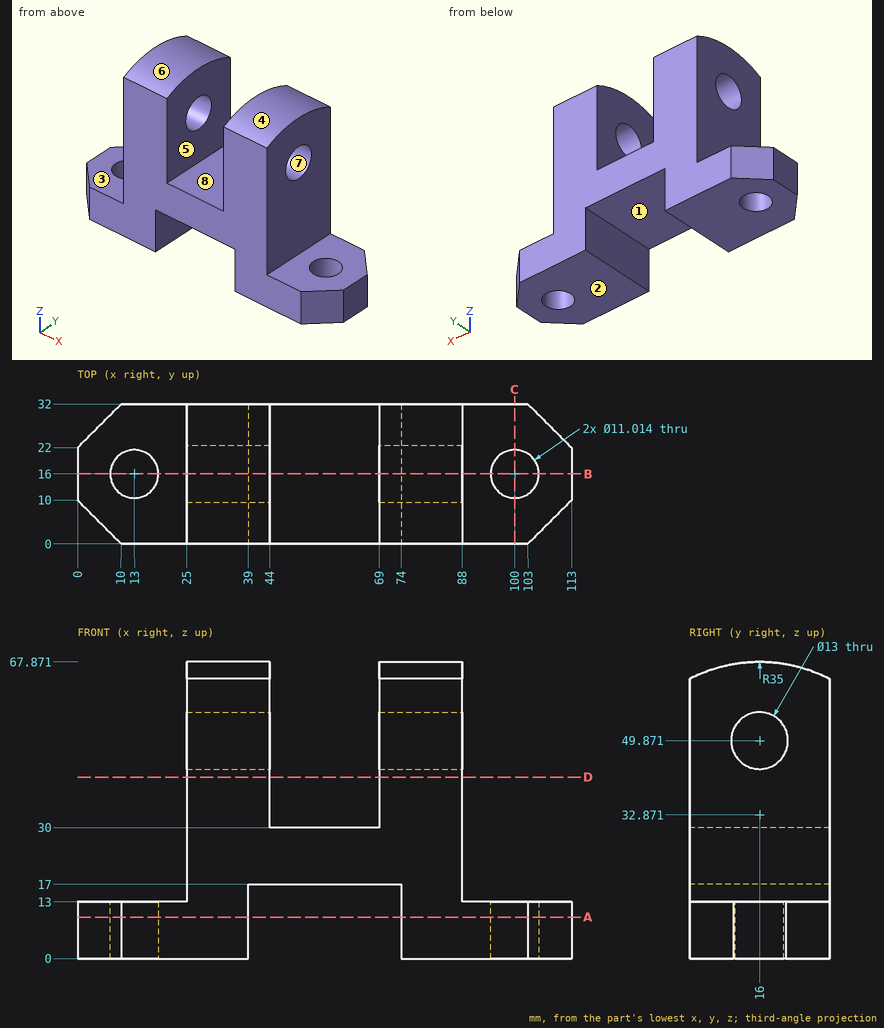
Geometry: see drawing. Coordinates: mm, zero at the bounding-box minimum. A direction names the side the tool comes from. Coordinates: 2 decimals unless noted, no trailing zeros. Write each loop counter-clockwise with the first axis right and the second up, starting at its lowest first coordinate (ties: lowest second). Pieces come first, ordered by that corner, then holes. Notation, with made-up numbers: M 40,-37 L 48,-37 A25 ccw 48,-19 Z; hole C 33.25,21 d10. An arc over 180 degrees is marked long. Answer as a JSON object with one key per item and string values.
1. Ray query, L1, parallel to Y at x = 100, z = 3.5; L2, parallel to X at y = 15, z = 15; L3, parallel to Z at x = 81.5, y = 16. Return the intervals inside material, ascending.
Evaluation:
{"L1": "0 to 10.49, 21.51 to 32", "L2": "25 to 39, 74 to 88", "L3": "0 to 43.37, 56.37 to 67.87"}
2. Cut plane C-C on x = 100. Output: boundary loops of the cut face in (y, z).
Evaluation:
{"outline": "M 0,0 L 10.49,0 L 10.49,13 L 0,13 Z; M 21.51,0 L 32,0 L 32,13 L 21.51,13 Z"}
3. Contact query for flat-ended pins moving along their axis: P1, Ø9.5, axis at y = 19.5, z = 46, coming from the +X side; P2, Ø12.5, axis at x = 55, y = 16.5, coming from the +Z side; P3, Ø6.5, axis at x = 13, y = 16, coming from the -Z side; P4, Ø6, axis at x = 91.5, y = 11.5, coming from the +Z side. Output: stop coordinate, or through.
Evaluation:
{"P1": "x = 88", "P2": "z = 30", "P3": "through", "P4": "z = 13"}
4. Draft query along Y for the marked faces 6, 7 and 8. Return one class per face: released by +Y, released by -Y, zero draft, split by the parting line, or undercut.
Evaluation:
{"face 6": "split by the parting line", "face 7": "undercut", "face 8": "zero draft"}
5. Cut plane D-D on z = 41.5. Output: boundary loops of the cut face in (x, y).
Evaluation:
{"outline": "M 25,0 L 44,0 L 44,32 L 25,32 Z; M 69,0 L 88,0 L 88,32 L 69,32 Z"}
6. Access query for the marked faces 1, 2, 3, 4 and 5. Directions: +Z, -Z, +X, -X, +Y, -Y. A direction counts if a zero-diameter tool reaches every point of the face in a straight line with its end or side. Return the directions, or none.
Evaluation:
{"face 1": "-Z, +Y, -Y", "face 2": "-Z, +X, -X, +Y, -Y", "face 3": "+Z, -X, +Y, -Y", "face 4": "+Z, +X, -X", "face 5": "+Z, +Y, -Y"}
7. Cut plane A-A on z = 9.5. Output: boundary loops of the cut face in (x, y).
Evaluation:
{"outline": "M 0,10 L 10,0 L 39,0 L 39,32 L 10,32 L 0,22 Z; M 74,0 L 103,0 L 113,10 L 113,22 L 103,32 L 74,32 Z; hole C 13,16 d11.01; hole C 100,16 d11.01"}
8. Cut plane B-B on y = 16. State how many separate pieces and enclosed holes the cut face has, plus the area to 3 significant figures.
Evaluation:
{"separate pieces": "5", "enclosed holes": "0", "area": "2,600 mm^2"}
